The listing builds one solid part. Answer for the finished solid, in the listing's coordinates (mm). A direction names the side the tool comes from. Round coordinates to 2 decimals unless told otherwise and drop trailing zeros. Loops run counter-clockwise (first coordinate to the right, second up) from the corner with the lowest first, then second, coordinate; pieces in that order, holes last. Notation, with made-up numbers: (86.5, -16.75) -> (109.5, -16.75) arc R21 cw to (109.5, -3.75) -> close; hole circle Ø7 at (45, -20.75). An arc over 180 degrees is marked (long way). Write each question's results on one line, items separated by ' | '. Start each with the question number.
(1) Straight lines are drawn through the part: probe 1 along Z at (x, y) = (0.25, 2.75); probe 2 along Z at (x, y) = (0.55, 3); probe 3 along Z at (x, y) = (0.4, -0.5). For each, find the intervals that lie inside material, in ascending order.
(2) The part is cut by section B-B (z = -2.25). Determine the outline of the cut face in (x, y).
(3) The part is cut by section C-C (y = 2.75). Determine the outline of the cut face in (x, z), plus the area to 3 significant figures.
(4) The part is cut by section A-A (y = 0). Determine the outline of the cut face in (x, z), plus the area to 3 significant figures.
(5) For faces 4 (the face through (0.6, 3, 0)), 5 (the face through (0.3, 2.49, -2.46)), determine the directions among +Z, -Z, +X, -X, +Y, -Y from which every point of the face is accessible in a straight line to the end or side of a thin tool.
(6) Determine the mould class of faces 1 (the face through (0.3, 2.46, 2.49)), 2 (the face through (0.296, 4.497, -0.169)), 3 (the face through (0, 3, 0)) for opening direction Z: released by +Z, released by -Z, zero draft, split by the parting line, or undercut.
(7) The part is cut by section D-D (x = 0.25). Determine the outline of the cut face in (y, z), plus the area to 3 significant figures.
```python
from build123d import *

# Parameters (mm, degrees)
ESQUISSE1_R             = 4.5
BASE_EXTRUSION_DEPTH    = 0.6
ENL_V_MAT_EXTRU_1_DEPTH = 7.392182726


with BuildPart() as part:
    # Esquisse1 → Base-Extrusion (new body)
    with BuildSketch(Plane(origin=(0, 0, 0), x_dir=(0, 0, -1), z_dir=(1, 0, 0))):
        Circle(ESQUISSE1_R)
    extrude(amount=BASE_EXTRUSION_DEPTH)

    # Esquisse2 → Enlèv. mat.-Extru.1 (cut, through all)
    with BuildSketch(Plane(origin=(0.6, 0, 0), x_dir=(0, 0, -1), z_dir=(1, 0, 0))):
        with BuildLine():
            Line((0.756460917, 2.382806514), (1.524293779, 3.150639376))
            ThreePointArc((1.524293779, 3.150639376), (2.474873734, 2.474873734), (3.150639376, 1.524293779))
            Line((3.150639376, 1.524293779), (2.382806514, 0.756460917))
            ThreePointArc((2.382806514, 0.756460917), (2.442354814, -0.533763022), (1.85, -1.681517172))
            Line((1.85, -1.681517172), (1.85, -3.681517172))
            Line((1.85, -3.681517172), (1.980710639, -4.040641702))
            ThreePointArc((1.980710639, -4.040641702), (0, -4.5), (-1.980710639, -4.040641702))
            Line((-1.980710639, -4.040641702), (-1.85, -3.681517172))
            Line((-1.85, -3.681517172), (-1.85, -1.681517172))
            ThreePointArc((-1.85, -1.681517172), (-2.442354814, -0.533763022), (-2.382806514, 0.756460917))
            Line((-2.382806514, 0.756460917), (-3.150639376, 1.524293779))
            ThreePointArc((-3.150639376, 1.524293779), (-2.474873734, 2.474873734), (-1.524293779, 3.150639376))
            Line((-1.524293779, 3.150639376), (-0.756460917, 2.382806514))
            ThreePointArc((-0.756460917, 2.382806514), (0, 2.5), (0.756460917, 2.382806514))
        make_face()
    extrude(amount=-ENL_V_MAT_EXTRU_1_DEPTH, mode=Mode.SUBTRACT)


solid = part.part
```
Checked values:
1) probe 1: z = -3.56 to -2.17, -1.12 to 1.12, 2.17 to 3.56 | probe 2: z = -3.35 to -1.8, -1.37 to 1.37, 1.8 to 3.35 | probe 3: z = -4.47 to -2.45, 2.45 to 4.47
2) outline: (0, -3.9) -> (0.6, -3.9) -> (0.6, -1.09) -> (0, -1.09) -> close; (0, 2.68) -> (0.6, 2.68) -> (0.6, 3.9) -> (0, 3.9) -> close
3) outline: (0, -3.56) -> (0.6, -3.56) -> (0.6, -2.17) -> (0, -2.17) -> close; (0, -1.12) -> (0.6, -1.12) -> (0.6, 1.12) -> (0, 1.12) -> close; (0, 2.17) -> (0.6, 2.17) -> (0.6, 3.56) -> (0, 3.56) -> close | area: 3.02 mm2
4) outline: (0, -4.5) -> (0.6, -4.5) -> (0.6, -2.5) -> (0, -2.5) -> close; (0, 2.5) -> (0.6, 2.5) -> (0.6, 4.5) -> (0, 4.5) -> close | area: 2.40 mm2
5) face 4: +Z, -Z, +X, +Y, -Y | face 5: +X, -X
6) face 1: undercut | face 2: split by the parting line | face 3: zero draft
7) outline: (-4.04, -1.98) arc R4.5 ccw (long way) to (-4.04, 1.98) -> (-3.68, 1.85) -> (-1.68, 1.85) arc R2.5 cw to (0.76, 2.38) -> (1.52, 3.15) arc R3.5 cw to (3.15, 1.52) -> (2.38, 0.76) arc R2.5 cw to (2.38, -0.76) -> (3.15, -1.52) arc R3.5 cw to (1.52, -3.15) -> (0.76, -2.38) arc R2.5 cw to (-1.68, -1.85) -> (-3.68, -1.85) -> close | area: 31.4 mm2
